```python
from build123d import *

# Parameters (mm, degrees)
BOSS_EXTRUDE1_DEPTH                = 76.2
SKETCH3_W                          = 34.29
SKETCH3_H                          = 76.2
BOSS_EXTRUDE2_DEPTH                = 63.5
FILLET1_R                          = 25.4
FILLET2_R                          = 25.4
F_1_3_4_5_TAPPED_HOLE1_D           = 39.6875
BOSS_EXTRUDE3_DEPTH                = 38.1
SKETCH10_W                         = 76.2
SKETCH10_H                         = 34.29
BOSS_EXTRUDE4_DEPTH                = 63.5
F_1_3_4_5_TAPPED_HOLE2_D           = 39.6875
F_1_3_4_5_TAPPED_HOLE2_CSINK_D     = 45.72
F_1_3_4_5_TAPPED_HOLE2_CSINK_ANGLE = 90


with BuildPart() as part:
    # Sketch2 → Boss-Extrude1 (new body)
    with BuildSketch(Plane(origin=(0, 0, 0), x_dir=(1, 0, 0), z_dir=(0, 1, 0))):
        Polygon((-101.6, -215.9), (-101.6, 241.3), (101.6, 241.3), (101.6, -215.9), (76.2, -215.9), (76.2, 215.9), (-76.2, 215.9), (-76.2, -215.9), align=None)
    extrude(amount=BOSS_EXTRUDE1_DEPTH)

    # Sketch3 → Boss-Extrude2 (add)
    with BuildSketch(Plane(origin=(101.6, 0, 0), x_dir=(0, 0, -1), z_dir=(1, 0, 0))):
        with Locations((-198.755, 38.1)):
            Rectangle(SKETCH3_W, SKETCH3_H)
    boss_extrude2 = extrude(amount=BOSS_EXTRUDE2_DEPTH)

    # Mirror1: Boss-Extrude2 across plane
    add(boss_extrude2.mirror(Plane(origin=(0, 0, 0), x_dir=(0, 0, 1), z_dir=(1, 0, 0))))

    # Fillet1
    fillet1_edges = [part.edges().sort_by_distance(p)[0] for p in [
        (-76.2, 38.1, 215.9),
        (-101.6, 38.1, -241.3),
        (101.6, 38.1, -241.3),
        (76.2, 38.1, 215.9),
    ]]
    fillet(fillet1_edges, radius=FILLET1_R)

    # Fillet2
    fillet2_edges = [part.edges().sort_by_distance(p)[0] for p in [
        (76.2, 38.1, -215.9),
        (-76.2, 38.1, -215.9),
    ]]
    fillet(fillet2_edges, radius=FILLET2_R)

    # 1-3/4-5 Tapped Hole1 (through all)
    with Locations(Plane(origin=(0, 0, 181.61), x_dir=(-1, 0, 0), z_dir=(0, 0, -1))):
        with Locations((-133.35, 38.1)):
            f_1_3_4_5_tapped_hole1 = Hole(F_1_3_4_5_TAPPED_HOLE1_D / 2)

    # Mirror2: 1-3/4-5 Tapped Hole1 across plane
    add(f_1_3_4_5_tapped_hole1.mirror(Plane(origin=(0, 0, 0), x_dir=(0, 0, 1), z_dir=(1, 0, 0))), mode=Mode.SUBTRACT)

    # Sketch9 → Boss-Extrude3 (add, symmetric)
    with BuildSketch(Plane(origin=(0, 0, 0), x_dir=(0, 0, -1), z_dir=(1, 0, 0))):
        Polygon((-215.9, -63.5), (241.3, -63.5), (241.3, 38.1), (215.9, 38.1), (215.9, -38.1), (-215.9, -38.1), align=None)
    extrude(amount=BOSS_EXTRUDE3_DEPTH, both=True)

    # Sketch10 → Boss-Extrude4 (add)
    with BuildSketch(Plane.XZ.offset(63.5)):
        with Locations((0, 198.755)):
            Rectangle(SKETCH10_W, SKETCH10_H)
    extrude(amount=BOSS_EXTRUDE4_DEPTH)

    # 1-3/4-5 Tapped Hole2 (through all)
    with Locations(Plane(origin=(0, 0, 181.61), x_dir=(-1, 0, 0), z_dir=(0, 0, -1))):
        with Locations((0, -95.221260733)):
            CounterSinkHole(F_1_3_4_5_TAPPED_HOLE2_D / 2, F_1_3_4_5_TAPPED_HOLE2_CSINK_D / 2, counter_sink_angle=F_1_3_4_5_TAPPED_HOLE2_CSINK_ANGLE)


solid = part.part
```
For this review, take the finished solid that the model builds, in its own axes (mm). A direction names the side the tool comes from. Round coordinates to 2 decimals unless told otherwise and drop trailing zeros. Write each loop counter-clockwise with the first axis right and the second up, starting at its lowest first coordinate (ties: lowest second). Pieces come first, ordered by that corner, then holes. Notation, with made-up numbers: (-26.5, 63) - (29.5, 63) arc R28 cw to (29.5, 101) - close; hole circle Ø8 at (-26.75, 65). An arc over 180 degrees is marked (long way). Put each result on its own line as item: value.
Q1. Mouldability with a two-part tool opening along Y and no side actions: class faces 5 (the face through (68.56, 38.63, -208.66)), 6 (the face through (10.75, -78.37, 184.48)), 7 (the face through (88, 0, 5)) as released by +Y, released by -Y, zero draft, split by the parting line, or undercut.
Solved:
face 5: zero draft
face 6: undercut
face 7: released by -Y
Q2. Machinability: for faces 1 (the face through (-38.1, -54, 3)), 2 (the face through (-154, 38, 181.61)), 3 (the face through (-83.84, 38.63, 208.66)), 4 (the face through (154, 38, 181.61)), which of the approach directions +Z, -Z, +X, -X, +Y, -Y give a long, thin tool a straight path to every point of the face, cutting with its end or side? Answer none if there is none.
Solved:
face 1: +Z, -Z, -X, -Y
face 2: -Z, -X, +Y, -Y
face 3: +Z, +Y, -Y
face 4: -Z, +X, +Y, -Y
Q3. Insertion check: pin 1 Ø4 at (x, z) = (-30.5, -138) entering from -Y; pin 2 Ø12 at (x, y) = (-36.5, -87.5) entering from -Z; pin 3 Ø10 at (y, z) = (35.5, -3) entering from +X. Each pin has a flat end and moves straight along its axis. Give the tip position at first contact, or say it passes through.
Solved:
pin 1: stops at y = -63.5
pin 2: stops at z = 181.61
pin 3: stops at x = 101.6
Q4. We need section B-B (y = 38.1). Give the boundary of the cut face in (x, z).
Solved:
outline: (-165.1, 181.61) - (-153.19, 181.61) - (-153.19, 215.9) - (-165.1, 215.9) - close; (-113.51, 181.61) - (-101.6, 181.61) - (-101.6, -215.9) arc R25.4 ccw to (-76.2, -241.3) - (76.2, -241.3) arc R25.4 ccw to (101.6, -215.9) - (101.6, 181.61) - (113.51, 181.61) - (113.51, 215.9) - (101.6, 215.9) arc R25.4 ccw to (76.2, 190.5) - (76.2, -190.5) arc R25.4 cw to (50.8, -215.9) - (-50.8, -215.9) arc R25.4 cw to (-76.2, -190.5) - (-76.2, 190.5) arc R25.4 ccw to (-101.6, 215.9) - (-113.51, 215.9) - close; (153.19, 181.61) - (165.1, 181.61) - (165.1, 215.9) - (153.19, 215.9) - close
Q5. We need section D-D (x = -133.35). Give the boundary of the cut face in (y, z).
Solved:
outline: (0, 181.61) - (18.26, 181.61) - (18.26, 215.9) - (0, 215.9) - close; (57.94, 181.61) - (76.2, 181.61) - (76.2, 215.9) - (57.94, 215.9) - close
Q6. We need section A-A (x = 0). Give the boundary of the cut face in (y, z), and give its area (3 significant figures).
Solved:
outline: (-127, 181.61) - (-118.08, 181.61) - (-115.07, 184.63) - (-115.07, 215.9) - (-127, 215.9) - close; (-75.38, 184.63) - (-72.36, 181.61) - (-63.5, 181.61) - (-63.5, -241.3) - (76.2, -241.3) - (76.2, -215.9) - (-38.1, -215.9) - (-38.1, 215.9) - (-75.38, 215.9) - close
area: 15,300 mm2
Q7. Wall thickness on probe 1 along X at (y, z) = (38, 190); probe 2 along X at (y, z) = (62, 48); probe 3 along Y at (x, z) = (0, 203.5): over which ranges is each line inside the solid? List them lowest first.
Solved:
probe 1: x = -165.1 to -153.19, -113.51 to -76.2, 76.2 to 113.51, 153.19 to 165.1
probe 2: x = -101.6 to -76.2, 76.2 to 101.6
probe 3: y = -127 to -115.07, -75.38 to -38.1
Q8. We need section C-C (z = -54). Give the boundary of the cut face in (x, y), and give its area (3 significant figures).
Solved:
outline: (-101.6, 0) - (-76.2, 0) - (-76.2, 76.2) - (-101.6, 76.2) - close; (-38.1, -63.5) - (38.1, -63.5) - (38.1, -38.1) - (-38.1, -38.1) - close; (76.2, 0) - (101.6, 0) - (101.6, 76.2) - (76.2, 76.2) - close
area: 5,810 mm2
